from build123d import *

# Parameters (mm, degrees)
SKETCH1_R               = 19.05
SKETCH1_R_2             = 13.97
BOSS_EXTRUDE1_DEPTH     = 266.7
SKETCH2_R               = 13.97
BOSS_EXTRUDE2_DEPTH     = 6.35
SKETCH3_R               = 2.2479
CUT_EXTRUDE1_DEPTH      = 3.54
CUT_EXTRUDE1_DEPTH_BACK = 36.56
SKETCH5_W               = 10.16
SKETCH5_H               = 76.2
SKETCH5_H_2             = 50.8
SKETCH5_H_3             = 63.5
CUT_EXTRUDE5_DEPTH      = 20.0500001
CUT_EXTRUDE5_DEPTH_BACK = 20.0500001
SKETCH8_W               = 10.16
SKETCH8_H               = 76.2
SKETCH8_H_2             = 50.8
SKETCH8_H_3             = 63.5
CUT_EXTRUDE6_DEPTH      = 20.050000101
CUT_EXTRUDE6_DEPTH_BACK = 20.050000101
SKETCH7_R               = 6.35
CUT_EXTRUDE4_DEPTH      = 7.3500001


with BuildPart() as part:
    # Sketch1 → Boss-Extrude1 (new body)
    with BuildSketch(Plane(origin=(0, 0, 0), x_dir=(1, 0, 0), z_dir=(0, 1, 0))):
        Circle(SKETCH1_R)
        Circle(SKETCH1_R_2, mode=Mode.SUBTRACT)
    extrude(amount=BOSS_EXTRUDE1_DEPTH)

    # Sketch2 → Boss-Extrude2 (add)
    with BuildSketch(Plane.XZ):
        Circle(SKETCH2_R)
    extrude(amount=-BOSS_EXTRUDE2_DEPTH)

    # Sketch3 → Cut-Extrude1 (cut, two sides)
    with BuildSketch(Plane.XY.offset(16.51)) as cut_extrude1_sk:
        with Locations((0, 101.6)):
            Circle(SKETCH3_R)
    extrude(amount=CUT_EXTRUDE1_DEPTH, mode=Mode.SUBTRACT)
    extrude(cut_extrude1_sk.sketch, amount=-CUT_EXTRUDE1_DEPTH_BACK, mode=Mode.SUBTRACT)

    # Sketch5 → Cut-Extrude5 (cut, two sides)
    with BuildSketch(Plane(origin=(0, 0, 0), x_dir=(0, 0, -1), z_dir=(1, 0, 0))) as cut_extrude5_sk:
        with Locations((0, 50.8)):
            Rectangle(SKETCH5_W, SKETCH5_H)
        with Locations((0, 139.7)):
            Rectangle(SKETCH5_W, SKETCH5_H_2)
        with Locations((0, 222.25)):
            Rectangle(SKETCH5_W, SKETCH5_H_3)
    extrude(amount=CUT_EXTRUDE5_DEPTH, mode=Mode.SUBTRACT)
    extrude(cut_extrude5_sk.sketch, amount=-CUT_EXTRUDE5_DEPTH_BACK, mode=Mode.SUBTRACT)

    # Sketch8 → Cut-Extrude6 (cut, two sides)
    with BuildSketch(Plane.XY) as cut_extrude6_sk:
        with Locations((0, 50.8)):
            Rectangle(SKETCH8_W, SKETCH8_H)
        with Locations((0, 139.7)):
            Rectangle(SKETCH8_W, SKETCH8_H_2)
        with Locations((0, 222.25)):
            Rectangle(SKETCH8_W, SKETCH8_H_3)
    extrude(amount=CUT_EXTRUDE6_DEPTH, mode=Mode.SUBTRACT)
    extrude(cut_extrude6_sk.sketch, amount=-CUT_EXTRUDE6_DEPTH_BACK, mode=Mode.SUBTRACT)

    # Sketch7 → Cut-Extrude4 (cut, through all)
    with BuildSketch(Plane(origin=(0, 6.35, 0), x_dir=(1, 0, 0), z_dir=(0, 1, 0))):
        Circle(SKETCH7_R)
    extrude(amount=-CUT_EXTRUDE4_DEPTH, mode=Mode.SUBTRACT)


solid = part.part
Work out the finished part from the listing and answer in its coordinate system (mm). A direction names the side the tool comes from. Coordinates: 2 decimals unless noted, no trailing zeros. Loops run counter-clockwise (first coordinate to the right, second up) from the corner with the lowest first, then second, coordinate; pieces in that order, holes last. Notation, with made-up numbers: (54.5, 81.5) -> (106.5, 81.5) arc R26 ccw to (106.5, 100.5) -> close; hole circle Ø10 at (84, 53.5). An arc over 180 degrees is marked (long way). Answer as CSV lines item,"result".
1) Flat-ended cylindrical pins translate along their axes: pin 1 (3 mm diameter, centred on x = -1, z = -17, fed in from -Y); pin 2 (1.6 mm diameter, centred on y = 150, z = -15.5, fed in from -X); pin 3 (8 mm diameter, centred on x = 2.5, y = 83.5, fed in from -Z); pin 4 (4.5 mm diameter, centred on y = 48.5, z = -14.5, fed in from -X). Find the tip coordinate at first contact, or state that the pin passes through.
A:
pin 1,"stops at y = 0"
pin 2,"stops at x = -12.12"
pin 3,"stops at z = -18.36"
pin 4,"stops at x = -14.59"
2) Straight lines are drawn through the part: probe 1 along Y at (x, z) = (14, 2.5); probe 2 along Y at (x, z) = (0, -17); probe 3 along X at (y, z) = (4.25, 0). For each, find the intervals that lie inside material, in ascending order.
A:
probe 1,"y = 0 to 12.7, 88.9 to 114.3, 165.1 to 190.5, 254 to 266.7"
probe 2,"y = 0 to 12.7, 88.9 to 99.35, 103.85 to 114.3, 165.1 to 190.5, 254 to 266.7"
probe 3,"x = -19.05 to -6.35, 6.35 to 19.05"
3) The part is cut by section A-A (y = 36.5). Give the vertices of the cut face in (x, z), and give its area (3 significant figures).
A:
outline,"(-18.36, -5.08) arc R19.05 ccw to (-5.08, -18.36) -> (-5.08, -13.01) arc R13.97 cw to (-13.01, -5.08) -> close; (-18.36, 5.08) -> (-13.01, 5.08) arc R13.97 cw to (-5.08, 13.01) -> (-5.08, 18.36) arc R19.05 ccw to start; (5.08, -18.36) arc R19.05 ccw to (18.36, -5.08) -> (13.01, -5.08) arc R13.97 cw to (5.08, -13.01) -> close; (5.08, 13.01) arc R13.97 cw to (13.01, 5.08) -> (18.36, 5.08) arc R19.05 ccw to (5.08, 18.36) -> close"
area,"317 mm²"
4) For faces 3 (the face through (-5, 0, 5)), 4 (the face through (16, 222, 5.08)), 5 (the face through (0, 165.1, 16)), determine the directions among +Z, -Z, +X, -X, +Y, -Y from which every point of the face is accessible in a straight line to the end or side of a thin tool.
A:
face 3,"+Z, -Z, +X, -X, -Y"
face 4,"+X, -X"
face 5,"+Z, -Z"
5) For a pull along X with two mould halves and no side action, classify faces 1 (the face through (-5.08, 50, 16)), 2 (the face through (-16, 254, 0)) as released by +X, released by -X, zero draft, split by the parting line, or undercut.
A:
face 1,"undercut"
face 2,"zero draft"
6) The part is cut by section C-C (y = 172). Give the vertices of the cut face in (x, z), and give its area (3 significant figures).
A:
outline,"circle Ø38.1 at (0, 0); hole circle Ø27.94 at (0, 0)"
area,"527 mm²"
7) The part is cut by section B-B (x = 0). State how many separate pieces and enclosed holes the cut face has, and give its area (3 significant figures).
A:
separate pieces,"10"
enclosed holes,"0"
area,"825 mm²"
